Answer from the drawing. Dimensions are ordinates in mm from the lowest x, y and z of the part. Give positions to 0.01 mm unless a question says otherwise; leave off trailing zeros. Write each loop counter-clockwise with the first axis right and the second up, starting at its lowest first coordinate (ties: lowest second). Pieces come first, ordered by that corner, then holes. Notation, with made-up numbers: (16, 78) -> (70, 78) arc R18 ccw to (70, 113) -> close; hole circle Ø8 at (89.5, 32). An arc over 180 degrees is marked (long way). Write item = value, one per line.
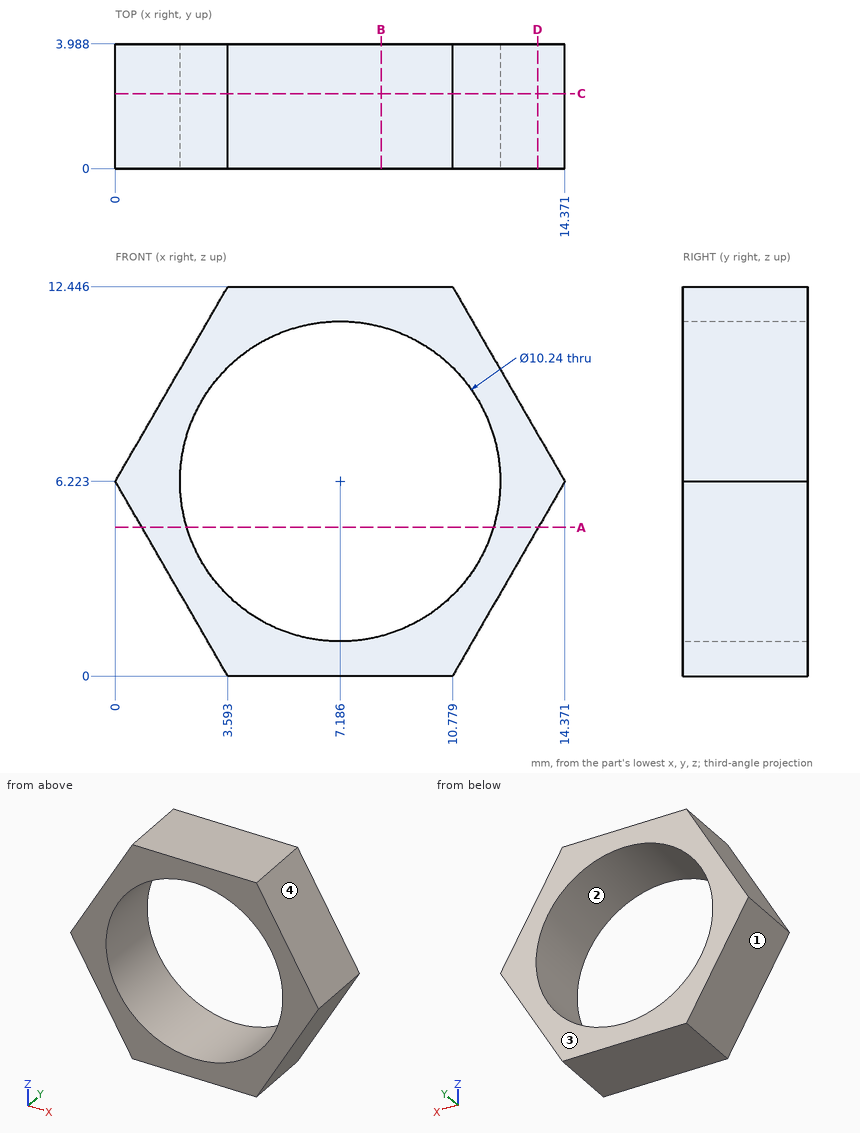
(1) The part is cut by section C-C on y = 2.4. Determine the outline of the cut face in (x, z) (1 decimal).
Checks:
outline = (0, 6.2) -> (3.6, 0) -> (10.8, 0) -> (14.4, 6.2) -> (10.8, 12.4) -> (3.6, 12.4) -> close; hole circle Ø10.2 at (7.2, 6.2)
(2) Given P1, Ø1.5, axis at x = 3.5, z = 5.5, coming from the -Y side, flat-ended and moving along its own axis, determine where the tip first touches the part or whether it passes through.
Checks:
P1 = through
(3) For a pull along X with two mould halves and no side action, classify the marked faces 1, 2, 3 and 4 as released by +X, released by -X, zero draft, split by the parting line, or undercut.
Checks:
face_1 = released by -X
face_2 = undercut
face_3 = zero draft
face_4 = released by +X
(4) The part is cut by section B-B on x = 8.5. Determine the outline of the cut face in (y, z) (1 decimal).
Checks:
outline = (0, 0) -> (4, 0) -> (4, 1.3) -> (0, 1.3) -> close; (0, 11.2) -> (4, 11.2) -> (4, 12.4) -> (0, 12.4) -> close
(5) The part is cut by section A-A on z = 4.75. Determine the outline of the cut face in (x, y), plus the area to 3 significant figures.
Checks:
outline = (0.85, 0) -> (2.28, 0) -> (2.28, 3.99) -> (0.85, 3.99) -> close; (12.09, 0) -> (13.52, 0) -> (13.52, 3.99) -> (12.09, 3.99) -> close
area = 11.4 mm²
(6) Consider L1, parallel to Z at x = 6.75, y = 1.9 (1 decimal); L2, parallel to Z at x = 11, y = 1.05 (1 decimal); L3, parallel to X at y = 0.65, z = 5 (1 decimal). Determine where each line is inside the solid, lowest interval first.
Checks:
L1 = 0 to 1.1, 11.3 to 12.4
L2 = 0.4 to 2.8, 9.6 to 12.1
L3 = 0.7 to 2.2, 12.2 to 13.7
(7) The part is cut by section D-D on x = 13.5. Determine the outline of the cut face in (y, z).
Checks:
outline = (0, 4.71) -> (3.99, 4.71) -> (3.99, 7.73) -> (0, 7.73) -> close
